```python
from build123d import *

# Parameters (mm, degrees)
SKETCH1_W           = 1340
SKETCH1_H           = 540
BOSS_EXTRUDE1_DEPTH = 100
SKETCH2_W           = 1280
SKETCH2_H           = 480
CUT_EXTRUDE1_DEPTH  = 80
SKETCH6_W           = 650
SKETCH6_H           = 600
BOSS_EXTRUDE3_DEPTH = 30
SKETCH10_R          = 2.5
CUT_EXTRUDE3_DEPTH  = 80
SKETCH11_R          = 4
CUT_EXTRUDE4_DEPTH  = 80


with BuildPart() as part:
    # Sketch1 → Boss-Extrude1 (new body)
    with BuildSketch(Plane(origin=(0, 0, 0), x_dir=(1, 0, 0), z_dir=(0, 1, 0))):
        Rectangle(SKETCH1_W, SKETCH1_H)
    extrude(amount=BOSS_EXTRUDE1_DEPTH)

    # Sketch2 → Cut-Extrude1 (cut)
    with BuildSketch(Plane(origin=(0, 100, 0), x_dir=(1, 0, 0), z_dir=(0, 1, 0))):
        Rectangle(SKETCH2_W, SKETCH2_H)
    extrude(amount=-CUT_EXTRUDE1_DEPTH, mode=Mode.SUBTRACT)

    # Sketch6 → Boss-Extrude3 (add)
    with BuildSketch(Plane(origin=(-640, 0, 0), x_dir=(0, 0, -1), z_dir=(1, 0, 0))):
        with Locations((0, -200)):
            Rectangle(SKETCH6_W, SKETCH6_H)
    boss_extrude3 = extrude(amount=-BOSS_EXTRUDE3_DEPTH)

    # Mirror3: Boss-Extrude3 across plane
    add(boss_extrude3.mirror(Plane(origin=(0, 0, 0), x_dir=(0, 0, 1), z_dir=(1, 0, 0))))

    # Sketch10 → Cut-Extrude3 (cut)
    with BuildSketch(Plane(origin=(-640, 0, 0), x_dir=(0, 0, -1), z_dir=(1, 0, 0))):
        with Locations((-160, 80)):
            Circle(SKETCH10_R)
        with Locations((-160, 42)):
            Circle(SKETCH10_R)
        with Locations((-80, 42)):
            Circle(SKETCH10_R)
        with Locations((-80, 80)):
            Circle(SKETCH10_R)
        with Locations((30, 80)):
            Circle(SKETCH10_R)
        with Locations((30, 42)):
            Circle(SKETCH10_R)
        with Locations((-8, 42)):
            Circle(SKETCH10_R)
        with Locations((-8, 80)):
            Circle(SKETCH10_R)
    cut_extrude3 = extrude(amount=-CUT_EXTRUDE3_DEPTH, mode=Mode.SUBTRACT)

    # Mirror4: Cut-Extrude3 across plane
    add(cut_extrude3.mirror(Plane(origin=(0, 0, 0), x_dir=(0, 0, 1), z_dir=(1, 0, 0))), mode=Mode.SUBTRACT)

    # Sketch11 → Cut-Extrude4 (cut)
    with BuildSketch(Plane(origin=(-640, 0, 0), x_dir=(0, 0, -1), z_dir=(1, 0, 0))):
        with Locations((-40, 61)):
            Circle(SKETCH11_R)
        with Locations((-120, 61)):
            Circle(SKETCH11_R)
    cut_extrude4 = extrude(amount=-CUT_EXTRUDE4_DEPTH, mode=Mode.SUBTRACT)

    # Mirror5: Cut-Extrude4 across plane
    add(cut_extrude4.mirror(Plane(origin=(0, 0, 0), x_dir=(0, 0, 1), z_dir=(1, 0, 0))), mode=Mode.SUBTRACT)


solid = part.part
```
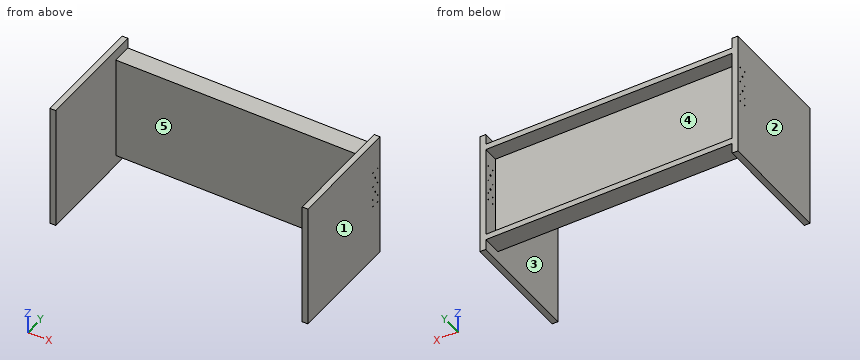
For this review, take the finished solid that the model builds, in its own axes (mm). Face numbers are marked on the shaded views. A direction names the side the tool comes from. Round coordinates to 2 decimals unless told otherwise and drop trailing zeros. Write each loop counter-clockwise with the first axis right and the second up, starting at its lowest first coordinate (ties: lowest second). Pieces come first, ordered by that corner, then holes. Notation, with made-up numbers: (66, 1.5) -> (114, 1.5) arc R24 cw to (114, 12.5) -> close; hole circle Ø10 at (34, 86). An arc over 180 degrees is marked (long way). Use one line per item in the form item = value.
Q1. The part is to be moulded in two halves that separate along X. For the marked faces 1, 2 and 3, say which applies: released by +X, released by -X, zero draft, split by the parting line, or undercut.
Resolved:
face_1 = released by +X
face_2 = released by -X
face_3 = undercut
Q2. To check wall thickness, follow probe 1 along Y at (x, z) = (-649.75, -30); probe 2 along Z at (x, y) = (646, 80); probe 3 along X at (y, z) = (-254.5, 97). State the ranges of each line that lie inside material, in increasing order. Write a range as from..to.
Resolved:
probe_1 = -500..39.5, 44.5..77.5, 82.5..100
probe_2 = -325..-32.5, -27.5..5.5, 10.5..77.5, 82.5..157.5, 162.5..325
probe_3 = -670..-640, 640..670
Q3. Consider section B-B (z = -283). State the section outline as (x, y) points, then the cut area to 3 significant figures.
Resolved:
outline = (-670, -500) -> (-640, -500) -> (-640, 100) -> (-670, 100) -> close; (640, -500) -> (670, -500) -> (670, 100) -> (640, 100) -> close
area = 36,000 mm²
Q4. Clearance check with flat-ended pins moving along their axes: pin 1 Ø12 at (x, z) = (-357.5, -54) entering from +Y; pin 2 Ø9 at (y, z) = (61, 40) entering from -X; pin 3 Ø6 at (x, z) = (444, -117.5) entering from -Y. State where each tip first meets the part, or that it passes through.
Resolved:
pin_1 = 20
pin_2 = -670
pin_3 = 0
Q5. Machinability: for the marked faces 4 and 5, which of the approach directions +Z, -Z, +X, -X, +Y, -Y give a long, thin tool a straight path to every point of the face, cutting with its end or side? Answer none if there is none.
Resolved:
face_4 = +Y
face_5 = +Z, -Z, -Y
Q6. Consider section D-D (z = -115). State the section outline as (x, y) points.
Resolved:
outline = (-670, -500) -> (-640, -500) -> (-640, 0) -> (640, 0) -> (640, -500) -> (670, -500) -> (670, 100) -> (640, 100) -> (640, 20) -> (-640, 20) -> (-640, 100) -> (-670, 100) -> close
Q7. Consider section A-A (y = -384.5). State the section outline as (x, z) points.
Resolved:
outline = (-670, -325) -> (-640, -325) -> (-640, 325) -> (-670, 325) -> close; (640, -325) -> (670, -325) -> (670, 325) -> (640, 325) -> close
Q8. Consider section C-C (x = -317). State the section outline as (y, z) points, then the cut area to 3 significant figures.
Resolved:
outline = (0, -270) -> (100, -270) -> (100, -240) -> (20, -240) -> (20, 240) -> (100, 240) -> (100, 270) -> (0, 270) -> close
area = 15,600 mm²
